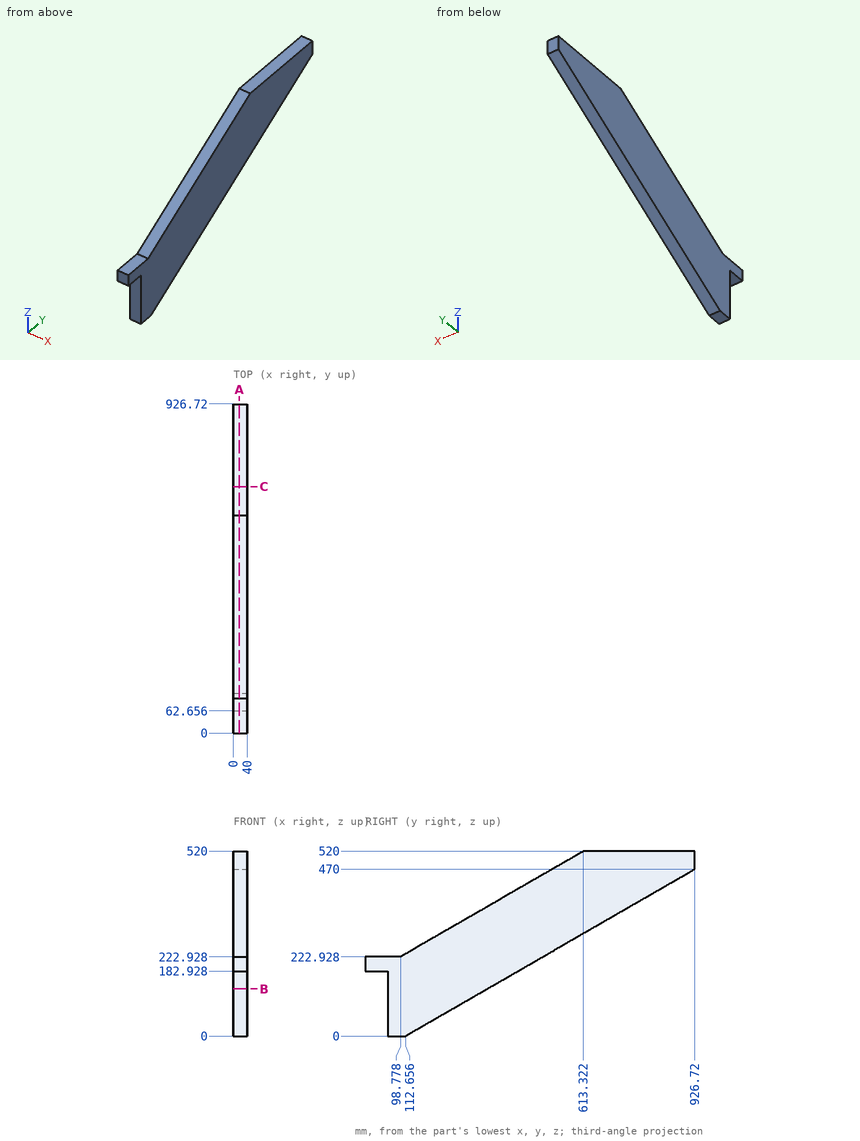
The figure shows three views and two pictorial views of one solid part (mm, origin at its lowest corner). Answer the questions. Round coordinates to 2 decimals unless told otherwise and drop trailing zeros. Loops run counter-clockwise (first coordinate to the right, second up) from the corner with the lowest first, then second, coordinate; pieces in that order, holes last. Notation, with made-up numbers: (9, 64) - (65, 64) arc R6 cw to (65, 68) - close; hole circle Ø8 at (-8, 50). An arc over 180 degrees is marked (long way). One line per question, with ' | ' between items. Start each with the question number.
Q1. Flat-ended cylindrical pins translate along their axes: pin 1 (12 mm diameter, centred on x = 18.5, y = 36, fed in from +Z); pin 2 (20 mm diameter, centred on x = 14.5, y = 34, fed in from -Z); pin 3 (2 mm diameter, centred on x = 7.5, z = 456, fed in from -Y). Find the tip coordinate at first contact, or state that the pin passes through.
Q2. Section B-B on z = 132.5 is taken. Give the vertices of the cut face in (x, y), plus the area to 3 significant figures.
Q3. Find the intervals of material crossed by L1, parallel to Y at x = 29.5, z = 202.5 (1 decimal); L2, parallel to Y at x = 38, z = 467 (1 decimal); L3, parallel to Z at x = 20, y = 170, in increasing order.
Q4. Section A-A on x = 17 is taken. Give the vertices of the cut face in (y, z), plus the area to 3 significant figures.
Q5. Section C-C on y = 694 is taken. Give the vertices of the cut face in (x, z), plus the area to 3 significant figures.
Established:
1) pin 1: z = 222.93 | pin 2: z = 182.93 | pin 3: y = 500.74
2) outline: (0, 62.66) - (40, 62.66) - (40, 342.15) - (0, 342.15) - close | area: 11,200 mm²
3) L1: 0 to 463.4 | L2: 521.5 to 921.5 | L3: 33.11 to 264.05
4) outline: (0, 182.93) - (62.66, 182.93) - (62.66, 0) - (112.66, 0) - (926.72, 470) - (926.72, 520) - (613.32, 520) - (98.78, 222.93) - (0, 222.93) - close | area: 173,000 mm²
5) outline: (0, 335.64) - (40, 335.64) - (40, 520) - (0, 520) - close | area: 7,370 mm²
